Input: part model. Units: mm. Frame: model coordinates. Face numbers are marked on the shaded views. A direction names the side the tool comes from. Coordinates: 2 decimals unless noted, no trailing zeros. Loops run counter-clockwise (first coordinate to the right, second up) from the corner with the lowest first, then second, coordinate; pieces in that order, holes last.
(1) Section A-A, the plane y = 0. Return loops of the section in (x, z).
(2) Section C-C, the plane z = 10.5. Return loops of the section in (x, y), then the cut area to 3 significant figures.
(3) Mould query, pull axis Z, two halves, no side actions, for the marked faces 3, 4, 5 and 6. Classes: released by +Z, released by -Z, zero draft, split by the parting line, or undercut.
(4) Contact query for flat-ended pins moving along their axis: P1, Ø4, axis at x = -12.5, z = 15.5, coming from the +Y side; P2, Ø12, axis at x = -15.5, z = 8.5, coming from the +Y side; P3, Ø8, axis at x = 13, z = 14.5, coming from the -Y side. Output: stop coordinate, or through.
(5) Set-up query: the marked faces 1 and 2. Return all of +Z, -Z, +X, -X, +Y, -Y with unobstructed straight access to the full face (end or side cutting, diameter ignored); none if empty.
(6) Section D-D, the plane z = 20. Return loops of the section in (x, y).
(7) Section B-B, the plane x = 0. Return loops of the section in (y, z).
(8) Line query: L1, parallel to Y at x = 0, z = 13.5; L2, parallel to Y at x = 0, z = 29; L3, parallel to Z at x = 1.5, y = -30. Output: solid intervals per line, ascending.
```python
from build123d import *

# Parameters (mm, degrees)
SKETCH1_R           = 32.5
BOSS_EXTRUDE1_DEPTH = 42
CUT_EXTRUDE1_START  = -28
SKETCH2_R           = 32.5
SKETCH2_R_2         = 30
CUT_EXTRUDE1_DEPTH  = 3
BOSS_EXTRUDE2_DEPTH = 14
FILLET1_R           = 2
CHAMFER1_SIZE       = 2
SKETCH4_R           = 21
CUT_EXTRUDE2_DEPTH  = 43


with BuildPart() as part:
    # Sketch1 → Boss-Extrude1 (new body)
    with BuildSketch(Plane.XY):
        Circle(SKETCH1_R)
    extrude(amount=BOSS_EXTRUDE1_DEPTH)

    # Sketch2 → Cut-Extrude1 (cut)
    with BuildSketch(Plane.XY.offset(42).offset(CUT_EXTRUDE1_START)):
        Circle(SKETCH2_R)
        Circle(SKETCH2_R_2, mode=Mode.SUBTRACT)
    extrude(amount=CUT_EXTRUDE1_DEPTH, mode=Mode.SUBTRACT)

    # Sketch3 → Boss-Extrude2 (add)
    with BuildSketch(Plane(origin=(0, 0, 0), x_dir=(-1, 0, 0), z_dir=(0, 0, -1))):
        Polygon((0, 37.527767497), (-32.5, 18.763883749), (-32.5, -18.763883749), (0, -37.527767497), (32.5, -18.763883749), (32.5, 18.763883749), align=None)
    extrude(amount=-BOSS_EXTRUDE2_DEPTH)

    # Fillet1
    fillet1_edges = [part.edges().sort_by_distance(p)[0] for p in [
        (0, 37.527767497, 7),
        (-32.5, 18.763883749, 7),
        (-32.5, -18.763883749, 7),
        (0, -37.527767497, 7),
        (32.5, -18.763883749, 7),
        (32.5, 18.763883749, 7),
    ]]
    fillet(fillet1_edges, radius=FILLET1_R)

    # Chamfer1
    chamfer1_edges = [part.edges().sort_by_distance(p)[0] for p in [
        (-32.5, 0, 42),
    ]]
    chamfer(chamfer1_edges, length=CHAMFER1_SIZE)

    # Sketch4 → Cut-Extrude2 (cut, through all)
    with BuildSketch(Plane.XY.offset(42)):
        Circle(SKETCH4_R)
    extrude(amount=-CUT_EXTRUDE2_DEPTH, mode=Mode.SUBTRACT)


solid = part.part
```
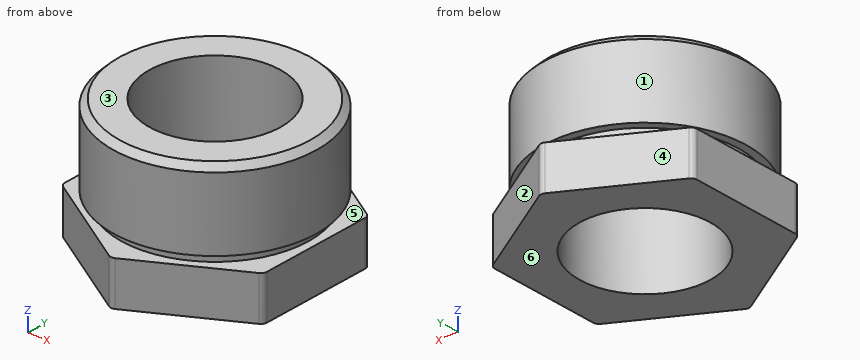
Report:
1. outline: (-32.5, 0) - (-21, 0) - (-21, 42) - (-30.5, 42) - (-32.5, 40) - (-32.5, 17) - (-30, 17) - (-30, 14) - (-32.5, 14) - close; (21, 0) - (32.5, 0) - (32.5, 14) - (30, 14) - (30, 17) - (32.5, 17) - (32.5, 40) - (30.5, 42) - (21, 42) - close
2. outline: (-32.5, -17.61) arc R2 ccw to (-31.5, -19.34) - (-1, -36.95) arc R2 ccw to (1, -36.95) - (31.5, -19.34) arc R2 ccw to (32.5, -17.61) - (32.5, 17.61) arc R2 ccw to (31.5, 19.34) - (1, 36.95) arc R2 ccw to (-1, 36.95) - (-31.5, 19.34) arc R2 ccw to (-32.5, 17.61) - close; hole circle Ø42 at (0, 0)
2. area: 2,270 mm2
3. face 3: released by +Z
3. face 4: zero draft
3. face 5: undercut
3. face 6: released by -Z
4. P1: stops at y = 31.07
4. P2: stops at y = 32.04
4. P3: stops at y = -32.31
5. face 1: +Z
5. face 2: +Z, -Z, +X, +Y
6. outline: circle Ø65 at (0, 0); hole circle Ø42 at (0, 0)
7. outline: (-37.22, 0) - (-21, 0) - (-21, 42) - (-30.5, 42) - (-32.5, 40) - (-32.5, 17) - (-30, 17) - (-30, 14) - (-37.22, 14) - close; (21, 0) - (37.22, 0) - (37.22, 14) - (30, 14) - (30, 17) - (32.5, 17) - (32.5, 40) - (30.5, 42) - (21, 42) - close
8. L1: y = -37.22 to -21, 21 to 37.22
8. L2: y = -32.5 to -21, 21 to 32.5
8. L3: z = 0 to 14, 17 to 42
